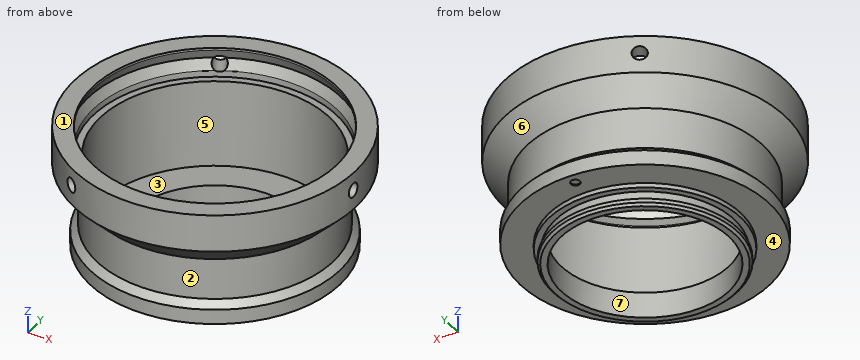
from build123d import *

# Parameters (mm, degrees)
ODEBRAT_START            = 25.986775
SKICA3_R                 = 1.5
ODEBRAT_VYSUNUT_M1_DEPTH = 4.013225
KRUHOV_POLE1_COUNT       = 3
SKICA4_R                 = 1
ODEBRAT_VYSUNUT_M2_DEPTH = 0.25


with BuildPart() as part:
    # Skica2 → Rotovat1 (revolve)
    with BuildSketch(Plane(origin=(0, 0, 0), x_dir=(0, 0, -1), z_dir=(1, 0, 0))):
        Polygon((-14.96, 17.955), (-14.96, 19.305), (-15.46, 19.805), (-16.3, 19.805), (-16.3, 19.155), (-18.3, 19.155), (-18.3, 20.5), (-19.3, 20.5), (-19.3, 26.67), (-22.45, 26.67), (-23.89, 25.23), (-32.69, 25.23), (-37.46, 30), (-45.46, 30), (-45.46, 26), (-44.96, 26), (-42.71, 27), (-40.46, 26), (-39.11, 26), (-39.11, 24.5), (-20.46, 24.5), (-20.46, 17.955), align=None)
    revolve(axis=Axis((0, 0, 0), (0, 0, 1)))

    # Skica3 → Odebrat vysunutím1 (cut)
    with BuildSketch(Plane(origin=(0, 0, 0), x_dir=(0, 0, -1), z_dir=(1, 0, 0)).offset(ODEBRAT_START)):
        with Locations((-41.71, 0)):
            Circle(SKICA3_R)
    odebrat_vysunut_m1 = extrude(amount=ODEBRAT_VYSUNUT_M1_DEPTH, mode=Mode.SUBTRACT)

    # Kruhové pole1: Odebrat vysunutím1 ×3 about axis
    kruhov_pole1_axis = Axis((0, 0, 0), (0, 0, -1))
    for i in range(1, KRUHOV_POLE1_COUNT):
        add(odebrat_vysunut_m1.rotate(kruhov_pole1_axis, i * 360 / KRUHOV_POLE1_COUNT), mode=Mode.SUBTRACT)

    # Skica4 → Odebrat vysunutím2 (cut)
    with BuildSketch(Plane(origin=(0, 0, 19.3), x_dir=(-1, 0, 0), z_dir=(0, 0, -1))):
        with Locations((0, 24.27)):
            Circle(SKICA4_R)
    extrude(amount=-ODEBRAT_VYSUNUT_M2_DEPTH, mode=Mode.SUBTRACT)


solid = part.part
For this review, take the finished solid that the model builds, in its own axes (mm). Face numbers are marked on the shaded views. A direction names the side the tool comes from. Give positions to 0.01 mm unless a question says otherwise; leave off trailing zeros. Order: outer loops, then holes, each group sorted by start corner. A loop starts at its lowest first (then second) coordinate and runs counter-clockwise, first axis right, second up. Notation, with made-up numbers: (80.5, 38) - (126.5, 38) arc R28 ccw to (126.5, 69) - close; hole circle Ø1 at (-34.5, 26.5). An arc over 180 degrees is marked (long way). Answer as a JSON object with one key per item and string values. Group by question number.
Item 1: Draft analysis for pull direction Y (two halves, no side actions). For the marked faces 4, 5, 6 and 7, state which applies: pulls with the +Y half, pulls with the -Y half, needs draft (parallel to the pull), parting line crosses it, or undercut.
Item 2: Take a section at A-A on z = 41.71. Give the boundary of the cut face in (x, y), and give its area (3 significant figures).
Item 3: Take a section at B-B on z = 28. Give the boundary of the cut face in (x, y), and give its area (3 significant figures).
Item 4: Wall thickness on line 1 along X through (y, z) = (0, 45.35); line 2 along Z through (x, y) = (19.5, 9): over which ranges is each line inside the solid? List them lowest first.
Item 5: Machinability: for the marked faces 1, 2 and 3, which of the approach directions +Z, -Z, +X, -X, +Y, -Y give a long, thin tool a straight path to every point of the face, cutting with its end or side? Answer none if there is none.
Item 6: Clearance check with flat-ended pins moving along their axes: pin 1 Ø10 at (y, z) = (21, 37.5) entering from +X; pin 2 Ø1.8 at (x, y) = (0, 24.27) entering from -Z; pin 3 Ø5 at (x, z) = (7, 21.5) entering from +Y; pin 4 Ø4 at (x, y) = (-4, -14.5) entering from -Z. State where each tip first meets the part, or that it passes through.
Item 7: Take a section at C-C on y = 0. Give the number of separate pieces and of enclosed holes in the cut face, and give its area (3 significant figures).
Reported:
{
 "1": {"face 4": "needs draft", "face 5": "undercut", "face 6": "parting line crosses it", "face 7": "undercut"},
 "2": {"outline": "(-16.28, -25.2) - (-14.56, -22.21) arc R26.56 cw to (-14.56, 22.21) - (-16.28, 25.2) arc R30 ccw to start; (-13.68, -26.7) arc R30 ccw to (29.96, -1.5) - (26.51, -1.5) arc R26.56 cw to (-11.96, -23.71) - close; (-13.68, 26.7) - (-11.96, 23.71) arc R26.56 cw to (26.51, 1.5) - (29.96, 1.5) arc R30 ccw to start", "area": "581 mm^2"},
 "3": {"outline": "circle Ø50.46 at (0, 0); hole circle Ø49 at (0, 0)", "area": "114 mm^2"},
 "4": {"line 1": "-30 to -26, 26 to 30", "line 2": "19.3 to 20.46"},
 "5": {"face 1": "+Z, +X, -X, +Y, -Y", "face 2": "none", "face 3": "+Z"},
 "6": {"pin 1": "x = 25.38", "pin 2": "z = 19.55", "pin 3": "y = 26.29", "pin 4": "through"},
 "7": {"separate pieces": "3", "enclosed holes": "0", "area": "144 mm^2"}
}
